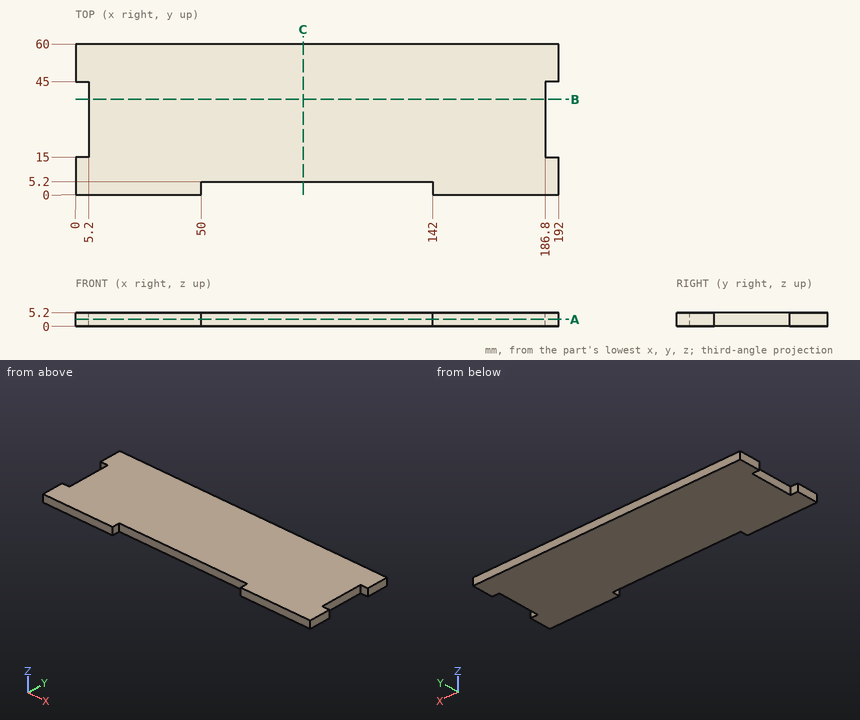
Study the drawing (mm; zero at the part's minimum x, y, z) and answer. Coordinates: 2 decimals unless noted, no trailing zeros. Loops run counter-clockwise (first coordinate to the right, second up) from the corner with the lowest first, then second, coordinate; pieces in that order, holes last. Notation, with made-up numbers: (63, 44) -> (105, 44) arc R21 ccw to (105, 52) -> close; hole circle Ø11 at (-38, -31.5). An arc over 180 degrees is marked (long way). Write item = value, one per line. Start each with the question number.
1) The part is cut by section A-A, the plane z = 2.65. Determine the outline of the cut face in (x, y).
2) The part is cut by section C-C, the plane x = 90.5. Determine the outline of the cut face in (y, z).
3) The part is cut by section B-B, the plane y = 38. Determine the outline of the cut face in (x, z).
4) Find the intervals of material crossed by L1, parallel to X at y = 5, z = 2.1; L2, parallel to X at y = 24.5, z = 3.6; L3, parallel to Y at x = 108, z = 3.1, in increasing order. Write a range as from..to.
5) Given P1, Ø2, axis at y = 26.5, z = 3, coming from the +X side; P2, Ø1.6, axis at y = 35.5, z = 3, coming from the -X side; P3, Ø3, axis at x = 70.5, z = 2.5, coming from the -Y side, each flat-ended and moving along its own axis, determine where each tip first touches the part or whether it passes through.
Result:
q1.outline = (0, 0) -> (50, 0) -> (50, 5.2) -> (142, 5.2) -> (142, 0) -> (192, 0) -> (192, 15) -> (186.8, 15) -> (186.8, 45) -> (192, 45) -> (192, 60) -> (0, 60) -> (0, 45) -> (5.2, 45) -> (5.2, 15) -> (0, 15) -> close
q2.outline = (5.2, 0) -> (60, 0) -> (60, 5.2) -> (5.2, 5.2) -> close
q3.outline = (5.2, 0) -> (186.8, 0) -> (186.8, 5.2) -> (5.2, 5.2) -> close
q4.L1 = 0..50, 142..192
q4.L2 = 5.2..186.8
q4.L3 = 5.2..60
q5.P1 = 186.8
q5.P2 = 5.2
q5.P3 = 5.2
